Here's how the part is built. I have some questions about the finished solid (model axes, mm). Coordinates: 2 decimals unless noted, no trailing zeros. Write each loop counter-clockwise with the first axis right and the second up, starting at its lowest first coordinate (ties: lowest second). Pieces come first, ordered by that corner, then holes.
Item 1: I want a section at B-B (x = 6). Please give me the cut outline in (y, z).
Item 2: If we mould it in two halves opening along Z, with no side actions, what happens to faces 1 (the face through (-18, 30, -4)), 2 (the face through (-25, 0, -6)), 3 (the face through (-18, 30, 3))? For each: pulls with the +Z half, pulls with the -Z half, needs draft (parallel to the pull), parting line crosses it, or undercut.
Item 3: I want a section at C-C (z = -25). Please give me the cut outline in (x, y), and give its area (3 significant figures).
Item 4: I'm going to push flat-ended pins straight in: P1, Ø4, axis at x = -4.5, y = 29, coming from the -Z side; P2, Ø2, axis at y = 31, z = -12, coming from the +X side; P3, Ø12, axis at y = 26, z = -10, coming from the +X side; P4, Ø1, axis at x = -43, z = -17, coming from the -Y side. Where does each tip first touch, or does it pass through?
Item 5: Please list where these lines run through material, in increasing order: line 1 (Z direction, x = 2, y = 7); line 2 (Z direction, x = -17, y = 53); line 3 (X direction, y = 21, z = -12).
Item 6: I want a section at A-A (y = 31). Please give me the cut outline in (x, z).
from build123d import *

# Parameters (mm, degrees)
BOSS_EXTRUDE1_DEPTH = 60
FILLET1_R           = 0.25


with BuildPart() as part:
    # Sketch1 → Boss-Extrude1 (new body)
    with BuildSketch(Plane(origin=(0, 0, 0), x_dir=(1, 0, 0), z_dir=(0, 1, 0))):
        Polygon((15, -3), (-15, -3), (-50.703700169, -3), (-50.703700169, 29), (-15, 4), (-20, 4), (-20, 3), (-15, 3), (15, 3), align=None)
    extrude(amount=BOSS_EXTRUDE1_DEPTH)

    # Fillet1
    fillet1_edges = [part.edges().sort_by_distance(p)[0] for p in [
        (-15, 30, -4),
    ]]
    fillet(fillet1_edges, radius=FILLET1_R)


solid = part.part
Answer:
1. outline: (0, -3) - (60, -3) - (60, 3) - (0, 3) - close
2. face 1: undercut
2. face 2: needs draft
2. face 3: pulls with the +Z half
3. outline: (-50.7, 0) - (-44.99, 0) - (-44.99, 60) - (-50.7, 60) - close
3. area: 343 mm2
4. P1: stops at z = -3
4. P2: stops at x = -25
4. P3: stops at x = -15.54
4. P4: stops at y = 0
5. line 1: z = -3 to 3
5. line 2: z = -5.4 to -4, -3 to 3
5. line 3: x = -50.7 to -26.43
6. outline: (-50.7, -29) - (-15.65, -4.45) arc R0.25 ccw to (-15.79, -4) - (-20, -4) - (-20, -3) - (15, -3) - (15, 3) - (-50.7, 3) - close
